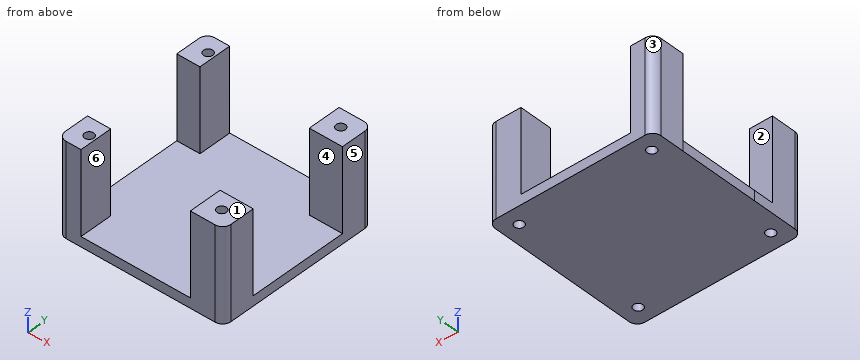
from build123d import *

# Parameters (mm, degrees)
SKETCH1_W           = 7.000000373
SKETCH1_H           = 6
SKETCH1_W_2         = 10.000000373
BOSS_EXTRUDE1_DEPTH = 3
SKETCH1_3_R         = 1.4
BOSS_EXTRUDE2_DEPTH = 28


with BuildPart() as part:
    # Sketch1 → Boss-Extrude1 (new body)
    with BuildSketch(Plane.XY):
        with Locations((-21.500000187, 12)):
            Rectangle(SKETCH1_W, SKETCH1_H)
        Polygon((25.000000373, -9), (25.000000373, 9), (15, 9), (15, 15), (15, 25.000000373), (-18, 25.000000373), (-18, 15), (-18, 9), (-25.000000373, 9), (-25.000000373, -9), (-18, -9), (-18, -15), (-18, -25.000000373), (15, -25.000000373), (15, -15), (15, -9), align=None)
        with Locations((20.000000187, -12)):
            Rectangle(SKETCH1_W_2, SKETCH1_H)
        with Locations((20.000000187, 12)):
            Rectangle(SKETCH1_W_2, SKETCH1_H)
        with Locations((-21.500000187, -12)):
            Rectangle(SKETCH1_W, SKETCH1_H)
    extrude(amount=BOSS_EXTRUDE1_DEPTH)

    # Sketch1_3 → Boss-Extrude2 (add)
    with BuildSketch(Plane.XY):
        with BuildLine():
            Line((-18, 25.000000373), (-22.500000373, 25.000000373))
            ThreePointArc((-22.500000373, 25.000000373), (-24.267767325, 24.267767325), (-25.000000373, 22.500000373))
            Line((-25.000000373, 22.500000373), (-25.000000373, 15))
            Line((-25.000000373, 15), (-18, 15))
            Line((-18, 15), (-18, 25.000000373))
        make_face()
        with Locations((-20, 20)):
            Circle(SKETCH1_3_R, mode=Mode.SUBTRACT)
        with BuildLine():
            Line((-25.000000373, -15), (-25.000000373, -22.500000373))
            ThreePointArc((-25.000000373, -22.500000373), (-24.267767325, -24.267767325), (-22.500000373, -25.000000373))
            Line((-22.500000373, -25.000000373), (-18, -25.000000373))
            Line((-18, -25.000000373), (-18, -15))
            Line((-18, -15), (-25.000000373, -15))
        make_face()
        with Locations((-20, -20)):
            Circle(SKETCH1_3_R, mode=Mode.SUBTRACT)
        with BuildLine():
            Line((25.000000373, 15), (25.000000373, 22.500000373))
            ThreePointArc((25.000000373, 22.500000373), (24.267767325, 24.267767325), (22.500000373, 25.000000373))
            Line((22.500000373, 25.000000373), (15, 25.000000373))
            Line((15, 25.000000373), (15, 15))
            Line((15, 15), (25.000000373, 15))
        make_face()
        with Locations((20, 20)):
            Circle(SKETCH1_3_R, mode=Mode.SUBTRACT)
        with BuildLine():
            Line((15, -25.000000373), (22.500000373, -25.000000373))
            ThreePointArc((22.500000373, -25.000000373), (24.267767325, -24.267767325), (25.000000373, -22.500000373))
            Line((25.000000373, -22.500000373), (25.000000373, -15))
            Line((25.000000373, -15), (15, -15))
            Line((15, -15), (15, -25.000000373))
        make_face()
        with Locations((20, -20)):
            Circle(SKETCH1_3_R, mode=Mode.SUBTRACT)
    extrude(amount=BOSS_EXTRUDE2_DEPTH)


solid = part.part
Check sheet for the modelled part. Datum: model origin and axes. Units: mm. Face numbers are marked on the shaded views. A direction names the side the tool comes from. Coordinates: 2 decimals unless noted, no trailing zeros. Write each loop counter-clockwise with the first axis right and the second up, starting at its lowest first coordinate (ties: lowest second). Pieces come first, ordered by that corner, then holes. Notation, with made-up numbers: M 73.25,-25 L 105.25,-25 A18 ccw 105.25,-9 Z; hole C -36,26.25 d7. An arc over 180 degrees is marked long. Answer as CSV lines item,"result".
Q1. Cross-section at B-B (x = 20). Record the boundary of the cut face in (y, z).
Check result:
outline,"M -25,0 L -21.4,0 L -21.4,28 L -25,28 Z; M -18.6,0 L 18.6,0 L 18.6,28 L 15,28 L 15,3 L -15,3 L -15,28 L -18.6,28 Z; M 21.4,0 L 25,0 L 25,28 L 21.4,28 Z"
Q2. Set-up check for the marked faces 4, 5 and 6: record each of +Z, -Z, +X, -X, +Y, -Y from which the full face is reachable in a straight line by a thin tool's end or side.
Check result:
face 4,"+Z, +X, -X"
face 5,"+Z, -Z, +X, +Y, -Y"
face 6,"+Z, +Y, -Y"
Q3. Cross-section at D-D (y = 7.5). Record the boundary of the cut face in (x, z), then the cut area to 3 significant figures.
Check result:
outline,"M -25,0 L 25,0 L 25,3 L -25,3 Z"
area,"150 mm^2"
Q4. Cross-section at C-C (y = 20). Record the boundary of the cut face in (x, z), then the cut area to 3 significant figures.
Check result:
outline,"M -25,0 L -21.4,0 L -21.4,28 L -25,28 Z; M -18.6,0 L 18.6,0 L 18.6,28 L 15,28 L 15,3 L -18,3 L -18,28 L -18.6,28 Z; M 21.4,0 L 25,0 L 25,28 L 21.4,28 Z"
area,"418 mm^2"
Q5. Mould release check, pull along Y, two halves, no side actions. Record for the marked faces 1, 2 and 3: released by +Y, released by -Y, zero draft, split by the parting line, or undercut.
Check result:
face 1,"zero draft"
face 2,"undercut"
face 3,"released by +Y"
Q6. Go/stop test with flat-tipped pins: pin 1 (2.5 mm diameter, centred on x = 20, y = -20, fed in from +Z); pin 2 (25 mm diameter, centred on x = -0.5, y = -7, fed in from +Z). Record where each tip stops, or that it passes through.
Check result:
pin 1,"through"
pin 2,"z = 3"
Q7. Cross-section at A-A (z = 20.25). Record the boundary of the cut face in (x, y).
Check result:
outline,"M -25,-22.5 A2.5 ccw -22.5,-25 L -18,-25 L -18,-15 L -25,-15 Z; M -25,15 L -18,15 L -18,25 L -22.5,25 A2.5 ccw -25,22.5 Z; M 15,-25 L 22.5,-25 A2.5 ccw 25,-22.5 L 25,-15 L 15,-15 Z; M 15,15 L 25,15 L 25,22.5 A2.5 ccw 22.5,25 L 15,25 Z; hole C -20,-20 d2.8; hole C -20,20 d2.8; hole C 20,-20 d2.8; hole C 20,20 d2.8"
Q8. Material ranges on probe 1 along Y at (x, z) = (-20, 20.5); probe 2 along X at (y, z) = (-17.5, 25); probe 3 along X at (y, z) = (19, 3.5), recorded low to high. Write a range as from..to.
Check result:
probe 1,"-25..-21.4, -18.6..-15, 15..18.6, 21.4..25"
probe 2,"-25..-18, 15..25"
probe 3,"-25..-20.98, -19.02..-18, 15..19.02, 20.98..25"
